Here's how the part is built. I have some questions about the finished solid (model axes, mm). Face numbers are marked on the shaded views. A direction names the side the tool comes from. Round coordinates to 2 decimals unless told otherwise and drop trailing zeros. Write each loop counter-clockwise with the first axis right and the second up, starting at its lowest first coordinate (ties: lowest second). Pieces come first, ordered by that corner, then holes. Notation, with made-up numbers: (71, -32) - (125, -32) arc R19 cw to (125, -19) - close; hole circle Ø9 at (25.25, 87.25). An arc over 180 degrees is marked (long way). One line per question, with ' | ' between items. Start each with the question number.
(1) Thinking about a two-plate mould opening in X: for the marked faces 1, 2, 3 and 4, which applies, pulls with the +X half, pulls with the -X half, needs draft (parallel to the pull), parting line crosses it, or undercut?
(2) Imagine slicing it at C-C (y = -15.5). Write out the boundary of the cut face in (x, z), plus the area to 3 significant figures.
(3) Imagine slicing it at B-B (z = 74.5). Write out the boundary of the cut face in (x, y), plus the area to 3 significant figures.
(4) If I drill on L1, parallel to Y at x = 25, z = 81; L2, parallel to X at y = -26, z = 30; L3, parallel to X at y = -33.5, z = 40.5, over which ranges is the centre line in solid material (lowest first)?
(5) For the marked faces 5 and 6, which set-ups out of +Z, -Z, +X, -X, +Y, -Y let a thin tool reach every point of the face, with its end or its side?
(6) Imagine slicing it at A-A (x = 17). Write out the boundary of the cut face in (y, z).
from build123d import *

# Parameters (mm, degrees)
F0_W         = 30
F0_H         = 30
F1_DEPTH     = 120
F2_R         = 1.5
F3_T1_DEPTH  = 30
F3_T3_DEPTH  = 30
F3_T6_ANGLE  = 90
F3_T8_ANGLE  = 90
F3_T10_ANGLE = 90
F3_T12_ANGLE = 90


# Not quite as in the source:
# - a fillet or chamfer that OpenCascade refuses, or shapes differently, is made with other operations: its cross-section is extruded or revolved along the edge and cut away or added


with BuildPart() as f1:
    # F0 (on Top) → F1 (new body)
    with BuildSketch(Plane.XY):
        with BuildLine():
            Line((33, 0), (3, 0))
            ThreePointArc((3, 0), (0.8786796564, -0.8786796564), (0, -3))
            Line((0, -3), (0, -33))
            ThreePointArc((0, -33), (0.8786796564, -35.1213203436), (3, -36))
            Line((3, -36), (33, -36))
            ThreePointArc((33, -36), (35.1213203436, -35.1213203436), (36, -33))
            Line((36, -33), (36, -3))
            ThreePointArc((36, -3), (35.1213203436, -0.8786796564), (33, 0))
        make_face()
        with Locations((18, -18)):
            Rectangle(F0_W, F0_H, mode=Mode.SUBTRACT)
    extrude(amount=F1_DEPTH)

    # F2
    f2_edges = [f1.edges().sort_by_distance(p)[0] for p in [
        (18, -33, 120),
        (3, -18, 120),
        (18, -3, 120),
        (33, -18, 120),
    ]]
    fillet(f2_edges, radius=F2_R)

    # F3: fillet of radius 1.5 on 4 edges, made by hand

    # F3_s2 → F3_t1 (cut)
    with BuildSketch(Plane.XZ.offset(3)):
        with BuildLine():
            ThreePointArc((34.5, 120), (35.5606601718, 119.5606601718), (36, 118.5))
            Line((36, 118.5), (36, 120))
            Line((36, 120), (34.5, 120))
        make_face()
        with BuildLine():
            ThreePointArc((1.5, 120), (0.4393398282, 119.5606601718), (0, 118.5))
            Line((0, 118.5), (0, 120))
            Line((0, 120), (1.5, 120))
        make_face()
    extrude(amount=F3_T1_DEPTH, mode=Mode.SUBTRACT)

    # F3_s4 → F3_t3 (cut)
    with BuildSketch(Plane.YZ.offset(3)):
        with BuildLine():
            ThreePointArc((-1.5, 120), (-0.4393398282, 119.5606601718), (0, 118.5))
            Line((0, 118.5), (0, 120))
            Line((0, 120), (-1.5, 120))
        make_face()
        with BuildLine():
            ThreePointArc((-34.5, 120), (-35.5606601718, 119.5606601718), (-36, 118.5))
            Line((-36, 118.5), (-36, 120))
            Line((-36, 120), (-34.5, 120))
        make_face()
    extrude(amount=F3_T3_DEPTH, mode=Mode.SUBTRACT)

    # F3_s5 → F3_t6 (revolve, cut)
    with BuildSketch(Plane.XZ.offset(3)):
        with BuildLine():
            ThreePointArc((34.5, 120), (35.5606601718, 119.5606601718), (36, 118.5))
            Line((36, 118.5), (36, 120))
            Line((36, 120), (34.5, 120))
        make_face()
    revolve(axis=Axis((33, -3, 120), (0, 0, 1)), revolution_arc=F3_T6_ANGLE, mode=Mode.SUBTRACT)

    # F3_s7 → F3_t8 (revolve, cut)
    with BuildSketch(Plane.YZ.offset(3)):
        with BuildLine():
            ThreePointArc((-1.5, 120), (-0.4393398282, 119.5606601718), (0, 118.5))
            Line((0, 118.5), (0, 120))
            Line((0, 120), (-1.5, 120))
        make_face()
    revolve(axis=Axis((3, -3, 120), (0, 0, 1)), revolution_arc=F3_T8_ANGLE, mode=Mode.SUBTRACT)

    # F3_s9 → F3_t10 (revolve, cut)
    with BuildSketch(Plane.XZ.offset(33)):
        with BuildLine():
            ThreePointArc((1.5, 120), (0.4393398282, 119.5606601718), (0, 118.5))
            Line((0, 118.5), (0, 120))
            Line((0, 120), (1.5, 120))
        make_face()
    revolve(axis=Axis((3, -33, 120), (0, 0, 1)), revolution_arc=F3_T10_ANGLE, mode=Mode.SUBTRACT)

    # F3_s11 → F3_t12 (revolve, cut)
    with BuildSketch(Plane.YZ.offset(33)):
        with BuildLine():
            ThreePointArc((-34.5, 120), (-35.5606601718, 119.5606601718), (-36, 118.5))
            Line((-36, 118.5), (-36, 120))
            Line((-36, 120), (-34.5, 120))
        make_face()
    revolve(axis=Axis((33, -33, 120), (0, 0, 1)), revolution_arc=F3_T12_ANGLE, mode=Mode.SUBTRACT)


solid = f1.part
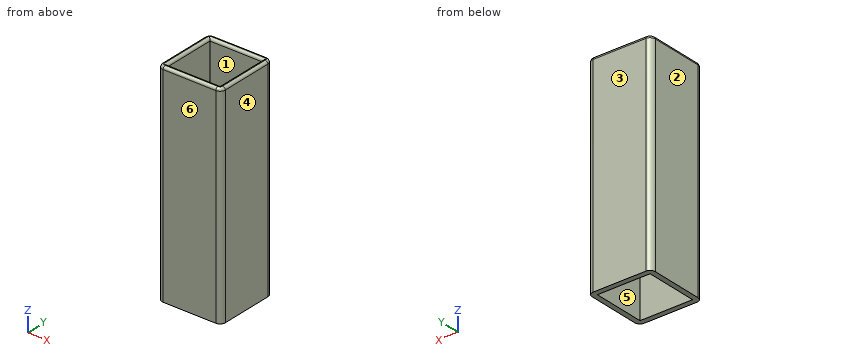
Check sheet entries:
1) face 1: undercut | face 2: pulls with the -X half | face 3: needs draft | face 4: pulls with the +X half
2) outline: (0, 0) - (3, 0) - (3, 118.5) arc R1.5 ccw to (0, 118.5) - close; (33, 0) - (36, 0) - (36, 118.5) arc R1.5 ccw to (33, 118.5) - close | area: 718 mm^2
3) outline: (0, -33) arc R3 ccw to (3, -36) - (33, -36) arc R3 ccw to (36, -33) - (36, -3) arc R3 ccw to (33, 0) - (3, 0) arc R3 ccw to (0, -3) - close; hole (3, -33) - (33, -33) - (33, -3) - (3, -3) - close | area: 388 mm^2
4) L1: -36 to -33, -3 to 0 | L2: 0 to 3, 33 to 36 | L3: 0.04 to 35.96
5) face 5: +Z, -Z | face 6: +Z, -Z, +X, -X, -Y
6) outline: (-36, 0) - (-33, 0) - (-33, 118.5) arc R1.5 ccw to (-36, 118.5) - close; (-3, 0) - (0, 0) - (0, 118.5) arc R1.5 ccw to (-3, 118.5) - close
